from build123d import *

# Parameters (mm, degrees)
SKETCH1_W           = 30
SKETCH1_H           = 30
BOSS_EXTRUDE1_DEPTH = 4
SKETCH2_R           = 2.1
CUT_EXTRUDE1_DEPTH  = 22.587033145
SKETCH3_R           = 10
BOSS_EXTRUDE2_DEPTH = 120
SKETCH4_2_W         = 40
SKETCH4_2_H         = 25
BOSS_EXTRUDE3_DEPTH = 3
SKETCH7_R           = 1.2
CUT_EXTRUDE2_DEPTH  = 30
CUT_EXTRUDE3_DEPTH  = 30


with BuildPart() as part:
    # Sketch1 → Boss-Extrude1 (new body)
    with BuildSketch(Plane(origin=(0, 0, 0), x_dir=(1, 0, 0), z_dir=(0, 1, 0))):
        Rectangle(SKETCH1_W, SKETCH1_H)
    extrude(amount=BOSS_EXTRUDE1_DEPTH)

    # Sketch2 → Cut-Extrude1 (cut, through all)
    with BuildSketch(Plane(origin=(0, 4, 0), x_dir=(1, 0, 0), z_dir=(0, 1, 0))):
        with Locations(Location((-10, 10, 0), (0, 0, 270))):
            Circle(SKETCH2_R)
        with Locations(Location((10, -10, 0), (0, 0, 270))):
            Circle(SKETCH2_R)
    extrude(amount=-CUT_EXTRUDE1_DEPTH, mode=Mode.SUBTRACT)

    # Sketch3 → Boss-Extrude2 (add)
    with BuildSketch(Plane(origin=(0, 4, 0), x_dir=(1, 0, 0), z_dir=(0, 1, 0))):
        with Locations(Location((0, 0, 0), (0, 0, 270))):
            Circle(SKETCH3_R)
    extrude(amount=BOSS_EXTRUDE2_DEPTH)

    # Sketch5 for Loft1 → Loft1 section 0
    with BuildSketch(Plane(origin=(0, 124, 0), x_dir=(1, 0, 0), z_dir=(0, 1, 0))):
        with BuildLine():
            # circular arc as an exact rational Bezier (weights 1, cos(half-angle), 1)
            Bezier((-8.47998304, -5.2999894), (0, -18.867962264), (8.47998304, -5.2999894), weights=[1, 0.52999894, 1])
            Bezier((8.47998304, -5.2999894), (11.792476415, 0), (8.47998304, 5.2999894), weights=[1, 0.847998304, 1])
            Bezier((8.47998304, 5.2999894), (0, 18.867962264), (-8.47998304, 5.2999894), weights=[1, 0.52999894, 1])
            Bezier((-8.47998304, 5.2999894), (-11.792476415, 0), (-8.47998304, -5.2999894), weights=[1, 0.847998304, 1])
        make_face()
    # Sketch4 → Loft1 section 1
    with BuildSketch(Plane(origin=(0, 144, 0), x_dir=(1, 0, 0), z_dir=(0, 1, 0))):
        with BuildLine():
            Line((-20, -12.5), (20, -12.5))
            Line((20, -12.5), (20, 12.5))
            Line((20, 12.5), (-20, 12.5))
            Line((-20, 12.5), (-20, -12.5))
        make_face()
    loft()

    # Sketch4_2 → Boss-Extrude3 (add)
    with BuildSketch(Plane(origin=(0, 144, 0), x_dir=(1, 0, 0), z_dir=(0, 1, 0))):
        Rectangle(SKETCH4_2_W, SKETCH4_2_H)
    extrude(amount=BOSS_EXTRUDE3_DEPTH)

    # Sketch7 → Cut-Extrude2 (cut)
    with BuildSketch(Plane(origin=(0, 147, 0), x_dir=(1, 0, 0), z_dir=(0, 1, 0))):
        with Locations(Location((-16.5, 8.75, 0), (0, 0, 270))):
            Circle(SKETCH7_R)
        with Locations(Location((-16.5, -8.75, 0), (0, 0, 270))):
            Circle(SKETCH7_R)
        with Locations(Location((16.5, 8.75, 0), (0, 0, 270))):
            Circle(SKETCH7_R)
        with Locations(Location((16.5, -8.75, 0), (0, 0, 270))):
            Circle(SKETCH7_R)
    extrude(amount=-CUT_EXTRUDE2_DEPTH, mode=Mode.SUBTRACT)

    # Sketch8 → Cut-Extrude3 (cut)
    with BuildSketch(Plane(origin=(0, 144, 0), x_dir=(1, 0, 0), z_dir=(0, 1, 0))):
        Polygon((-17.683568052, 6.7), (-15.316431948, 6.7), (-14.132863896, 8.75), (-15.316431948, 10.8), (-17.683568052, 10.8), (-18.867136104, 8.75), align=None)
        Polygon((-15.316431948, -6.7), (-17.683568052, -6.7), (-18.867136104, -8.75), (-17.683568052, -10.8), (-15.316431948, -10.8), (-14.132863896, -8.75), align=None)
        Polygon((15.316431948, 6.7), (17.683568052, 6.7), (18.867136104, 8.75), (17.683568052, 10.8), (15.316431948, 10.8), (14.132863896, 8.75), align=None)
        Polygon((14.132863896, -8.75), (15.316431948, -10.8), (17.683568052, -10.8), (18.867136104, -8.75), (17.683568052, -6.7), (15.316431948, -6.7), align=None)
    extrude(amount=-CUT_EXTRUDE3_DEPTH, mode=Mode.SUBTRACT)


solid = part.part
Design review of the part built by this model. Coordinates are the model's own, in mm. A direction names the side the tool comes from. Coordinates: 2 decimals unless noted, no trailing zeros. Write each loop counter-clockwise with the first axis right and the second up, starting at its lowest first coordinate (ties: lowest second). Pieces come first, ordered by that corner, then holes. Notation, with made-up numbers: (24.5, 36) -> (32.5, 36) arc R34 cw to (32.5, 75) -> close; hole circle Ø6 at (69.5, 49). An arc over 180 degrees is marked (long way). Write each question's results on one line, items separated by ' | '. Start each with the question number.
(1) Take a section at A-A on y = 85.5. Write out the cut boundary in (x, z).
(2) Tool access review of faces 1 (the face through (-9.76, 63.16, -2.17)), 2 (the face through (15, 2, 0)), 3 (the face through (-15, 2, 0)), 4 (the face through (-20, 145, 0)), 5 (the face through (-16, 141, 6.7)): name each direction out of +Z, -Z, +X, -X, +Y, -Y from which nothing blocks a thin tool from reaching the whole face with its end or side.
(3) The part is to be moulded in two halves that separate along Y. For faces 6 (the face through (0, 147, 0)), 7 (the face through (-15, 144, -8)), 8 (the face through (0, 145, 12.5)), 9 (the face through (-15, 144, 8)), say which applies: pulls with the +Y half, pulls with the -Y half, needs draft (parallel to the pull), parting line crosses it, or undercut.
(4) Clearance check with flat-ended pins moving along their axes: P1, Ø1.2, axis at x = -16, y = 138, coming from the -Z side; P2, Ø2.5, axis at x = 16, y = 139.5, coming from the -Z side; P3, Ø6, axis at x = 4.5, y = 21.5, coming from the +Z side; P4, Ø1.4, axis at x = -16.5, z = -8.75, coming from the +Y side. State where each tip first meets the part, or that it passes through.
(5) For line 1 along X through (y, z) = (146.25, 8.75); line 2 along Z through (x, y) = (-16, 145); line 3 along X through (y, z) = (1.2, 10), list the stretches that pass through material, from the lowest coordinate up. Write a range as from..to.
Results found:
1) outline: circle Ø20 at (0, 0)
2) face 1: none | face 2: +Z, -Z, +X, -Y | face 3: +Z, -Z, -X, -Y | face 4: +Z, -Z, -X, +Y, -Y | face 5: -Y
3) face 6: pulls with the +Y half | face 7: undercut | face 8: needs draft | face 9: undercut
4) P1: stops at z = -6.7 | P2: stops at z = -11.48 | P3: stops at z = 9.89 | P4: passes through
5) line 1: x = -20..-17.7, -15.3..15.3, 17.7..20 | line 2: z = -12.5..-9.84, -7.66..7.66, 9.84..12.5 | line 3: x = -15..7.9, 12.1..15
